from build123d import *

# Parameters (mm, degrees)
F0_R     = 2.5
F0_R_2   = 1.25
F1_DEPTH = 1.5
F2_DEPTH = 15
F3_DEPTH = 10
F5_W     = 13
F5_H     = 1.5
F6_DEPTH = 5


# Not quite as in the source:
# - a fillet or chamfer that OpenCascade refuses, or shapes differently, is made with other operations: its cross-section is extruded or revolved along the edge and cut away or added


with BuildPart() as f1:
    # F0 (on Top) → F1 (new body)
    with BuildSketch(Plane.XY):
        with BuildLine():
            ThreePointArc((26.5, -28), (27.2071067812, -27.7071067812), (27.5, -27))
            Line((27.5, -27), (27.5, 27))
            ThreePointArc((27.5, 27), (27.2071067812, 27.7071067812), (26.5, 28))
            Line((26.5, 28), (-26.5, 28))
            ThreePointArc((-26.5, 28), (-27.2071067812, 27.7071067812), (-27.5, 27))
            Line((-27.5, 27), (-27.5, -27))
            ThreePointArc((-27.5, -27), (-27.2071067812, -27.7071067812), (-26.5, -28))
            Line((-26.5, -28), (26.5, -28))
        make_face()
        with BuildLine():
            ThreePointArc((25.5, -25), (25.2071067812, -25.7071067812), (24.5, -26))
            Line((24.5, -26), (-24.5, -26))
            ThreePointArc((-24.5, -26), (-25.2071067812, -25.7071067812), (-25.5, -25))
            Line((-25.5, -25), (-25.5, 25))
            ThreePointArc((-25.5, 25), (-25.2071067812, 25.7071067812), (-24.5, 26))
            Line((-24.5, 26), (24.5, 26))
            ThreePointArc((24.5, 26), (25.2071067812, 25.7071067812), (25.5, 25))
            Line((25.5, 25), (25.5, -25))
        make_face(mode=Mode.SUBTRACT)
        with BuildLine():
            Line((-24.5, -26), (24.5, -26))
            ThreePointArc((24.5, -26), (25.2071067812, -25.7071067812), (25.5, -25))
            Line((25.5, -25), (25.5, 25))
            ThreePointArc((25.5, 25), (25.2071067812, 25.7071067812), (24.5, 26))
            Line((24.5, 26), (-24.5, 26))
            ThreePointArc((-24.5, 26), (-25.2071067812, 25.7071067812), (-25.5, 25))
            Line((-25.5, 25), (-25.5, -25))
            ThreePointArc((-25.5, -25), (-25.2071067812, -25.7071067812), (-24.5, -26))
        make_face()
        with Locations((-22, -22.5)):
            Circle(F0_R, mode=Mode.SUBTRACT)
        with Locations((22, -22.5)):
            Circle(F0_R, mode=Mode.SUBTRACT)
        with Locations((-22, 22.5)):
            Circle(F0_R, mode=Mode.SUBTRACT)
        with Locations((22, 22.5)):
            Circle(F0_R, mode=Mode.SUBTRACT)
        with Locations((-22, -22.5)):
            Circle(F0_R)
        with Locations((-22, -22.5)):
            Circle(F0_R_2, mode=Mode.SUBTRACT)
        with Locations((22, -22.5)):
            Circle(F0_R)
        with Locations((22, -22.5)):
            Circle(F0_R_2, mode=Mode.SUBTRACT)
        with Locations((22, 22.5)):
            Circle(F0_R)
        with Locations((22, 22.5)):
            Circle(F0_R_2, mode=Mode.SUBTRACT)
        with Locations((-22, 22.5)):
            Circle(F0_R)
        with Locations((-22, 22.5)):
            Circle(F0_R_2, mode=Mode.SUBTRACT)
        with Locations((-22, -22.5)):
            Circle(F0_R_2)
        with Locations((22, -22.5)):
            Circle(F0_R_2)
        with Locations((22, 22.5)):
            Circle(F0_R_2)
        with Locations((-22, 22.5)):
            Circle(F0_R_2)
    extrude(amount=F1_DEPTH)

    # F0 (on Top) → F2 (join)
    with BuildSketch(Plane.XY):
        with BuildLine():
            ThreePointArc((26.5, -28), (27.2071067812, -27.7071067812), (27.5, -27))
            Line((27.5, -27), (27.5, 27))
            ThreePointArc((27.5, 27), (27.2071067812, 27.7071067812), (26.5, 28))
            Line((26.5, 28), (-26.5, 28))
            ThreePointArc((-26.5, 28), (-27.2071067812, 27.7071067812), (-27.5, 27))
            Line((-27.5, 27), (-27.5, -27))
            ThreePointArc((-27.5, -27), (-27.2071067812, -27.7071067812), (-26.5, -28))
            Line((-26.5, -28), (26.5, -28))
        make_face()
        with BuildLine():
            ThreePointArc((25.5, -25), (25.2071067812, -25.7071067812), (24.5, -26))
            Line((24.5, -26), (-24.5, -26))
            ThreePointArc((-24.5, -26), (-25.2071067812, -25.7071067812), (-25.5, -25))
            Line((-25.5, -25), (-25.5, 25))
            ThreePointArc((-25.5, 25), (-25.2071067812, 25.7071067812), (-24.5, 26))
            Line((-24.5, 26), (24.5, 26))
            ThreePointArc((24.5, 26), (25.2071067812, 25.7071067812), (25.5, 25))
            Line((25.5, 25), (25.5, -25))
        make_face(mode=Mode.SUBTRACT)
    extrude(amount=F2_DEPTH)

    # F0 (on Top) → F3 (join)
    with BuildSketch(Plane.XY):
        with Locations((22, 22.5)):
            Circle(F0_R)
        with Locations((22, 22.5)):
            Circle(F0_R_2, mode=Mode.SUBTRACT)
        with Locations((-22, 22.5)):
            Circle(F0_R)
        with Locations((-22, 22.5)):
            Circle(F0_R_2, mode=Mode.SUBTRACT)
        with Locations((-22, -22.5)):
            Circle(F0_R)
        with Locations((-22, -22.5)):
            Circle(F0_R_2, mode=Mode.SUBTRACT)
        with Locations((22, -22.5)):
            Circle(F0_R)
        with Locations((22, -22.5)):
            Circle(F0_R_2, mode=Mode.SUBTRACT)
    extrude(amount=F3_DEPTH)

    # F4: fillet of radius 3 on 4 edges, made by hand

    # F4_s1 → F4_t2 (revolve)
    with BuildSketch(Plane.XZ.offset(22.5)):
        with BuildLine():
            ThreePointArc((27.5, 1.5), (25.3786796564, 2.3786796564), (24.5, 4.5))
            Line((24.5, 4.5), (24.5, 1.5))
            Line((24.5, 1.5), (27.5, 1.5))
        make_face()
    revolve(axis=Axis((22, -22.5, 1.5), (0, 0, -1)))

    # F4_s3 → F4_t4 (revolve)
    with BuildSketch(Plane.XZ.offset(-22.5)):
        with BuildLine():
            ThreePointArc((-16.5, 1.5), (-18.6213203436, 2.3786796564), (-19.5, 4.5))
            Line((-19.5, 4.5), (-19.5, 1.5))
            Line((-19.5, 1.5), (-16.5, 1.5))
        make_face()
    revolve(axis=Axis((-22, 22.5, 1.5), (0, 0, -1)))

    # F4_s5 → F4_t6 (revolve)
    with BuildSketch(Plane.XZ.offset(22.5)):
        with BuildLine():
            ThreePointArc((-16.5, 1.5), (-18.6213203436, 2.3786796564), (-19.5, 4.5))
            Line((-19.5, 4.5), (-19.5, 1.5))
            Line((-19.5, 1.5), (-16.5, 1.5))
        make_face()
    revolve(axis=Axis((-22, -22.5, 1.5), (0, 0, -1)))

    # F4_s7 → F4_t8 (revolve)
    with BuildSketch(Plane.XZ.offset(-22.5)):
        with BuildLine():
            ThreePointArc((27.5, 1.5), (25.3786796564, 2.3786796564), (24.5, 4.5))
            Line((24.5, 4.5), (24.5, 1.5))
            Line((24.5, 1.5), (27.5, 1.5))
        make_face()
    revolve(axis=Axis((22, 22.5, 1.5), (0, 0, -1)))

    # F5 (on face) → F6 (cut)
    with BuildSketch(Plane.XZ.offset(28)):
        with Locations((0, 2.4238943588)):
            Rectangle(F5_W, F5_H)
    extrude(amount=-F6_DEPTH, mode=Mode.SUBTRACT)


solid = f1.part
Part model, mm, in its own coordinate system. A direction names the side the tool comes from. Give positions to 0.01 mm unless a question says otherwise; leave off trailing zeros. Order: outer loops, then holes, each group sorted by start corner. A loop starts at its lowest first (then second) coordinate and runs counter-clockwise, first axis right, second up. Notation, with made-up numbers: (-22, 29) - (7, 29) arc R26 cw to (7, 51) - close; hole circle Ø8 at (34.25, 0.5). An arc over 180 degrees is marked (long way). Use a Markdown table: item, result.
1) Two-plate mould, pull along Z, no slides. Class faces 4 (the flat face through (23, -21, 10)), 5 (the flat face through (0, -27, 3.174)), 6 (the cylindrical face through (-20.845, -22.979, 5.69)): +Z half, -Z half, draft (parallel to the pull), parting line (faces both ways), or undercut.
Checked values:
| item | result |
|---|---|
| face 4 | +Z half |
| face 5 | undercut |
| face 6 | draft |
2) Saw through at B-B on y = -13.5. List the corners of the cut face in (x, z).
Checked values:
| item | result |
|---|---|
| outline | (-27.5, 0) - (27.5, 0) - (27.5, 15) - (25.5, 15) - (25.5, 1.5) - (-25.5, 1.5) - (-25.5, 15) - (-27.5, 15) - close |
3) Saw through at D-D on x = 10. List the corners of the cut face in (y, z).
Checked values:
| item | result |
|---|---|
| outline | (-28, 0) - (28, 0) - (28, 15) - (26, 15) - (26, 1.5) - (-26, 1.5) - (-26, 15) - (-28, 15) - close |
4) Flat gauge pins, fed straight in: P1, Ø3, axis at x = 8.5, y = -4, coming from the +Z side; P2, Ø4, axis at x = -22.5, y = -22, coming from the +Z side; P3, Ø1.2, axis at y = -27.5, z = 2.5, coming from the -X side. Where does each tip first touch, or does it go through?
Checked values:
| item | result |
|---|---|
| P1 | z = 1.5 |
| P2 | z = 10 |
| P3 | x = -27.5 |
5) 3-axis set-ups, long thin cutter, end or side, ignore diameter. For faces 1 (the cylindrical face through (23.155, 22.021, 5.69)), 2 (the flat face through (6.5, -27, 2)), 3 (the flat face through (-27, 0, 15)): which of +Z, -Z, +X, -X, +Y, -Y reach the whole face in a straight line?
Checked values:
| item | result |
|---|---|
| face 1 | +Z |
| face 2 | -Y |
| face 3 | +Z, +X, -X, +Y, -Y |
6) Saw through at A-A on z = 6. Count the separate pieces of the cut face and the enclosed holes in it, plus the area to 3 significant figures.
Checked values:
| item | result |
|---|---|
| separate pieces | 5 |
| enclosed holes | 5 |
| area | 487 mm² |
7) Probe L1, parallel to Y at x = 22, z = 8; L2, parallel to X at y = 22.5, z = 8; L3, parallel to X at y = 6.5, z = 4. List the from-to ranges inside material, lowest first. Write a range as from..to.
Checked values:
| item | result |
|---|---|
| L1 | -28..-26, -25..-23.75, -21.25..-20, 20..21.25, 23.75..25, 26..28 |
| L2 | -27.5..-25.5, -24.5..-23.25, -20.75..-19.5, 19.5..20.75, 23.25..24.5, 25.5..27.5 |
| L3 | -27.5..-25.5, 25.5..27.5 |
8) Saw through at C-C on z = 12. List the corners of the cut face in (x, y).
Checked values:
| item | result |
|---|---|
| outline | (-27.5, -27) arc R1 ccw to (-26.5, -28) - (26.5, -28) arc R1 ccw to (27.5, -27) - (27.5, 27) arc R1 ccw to (26.5, 28) - (-26.5, 28) arc R1 ccw to (-27.5, 27) - close; hole (-25.5, -25) arc R1 ccw to (-24.5, -26) - (24.5, -26) arc R1 ccw to (25.5, -25) - (25.5, 25) arc R1 ccw to (24.5, 26) - (-24.5, 26) arc R1 ccw to (-25.5, 25) - close |
